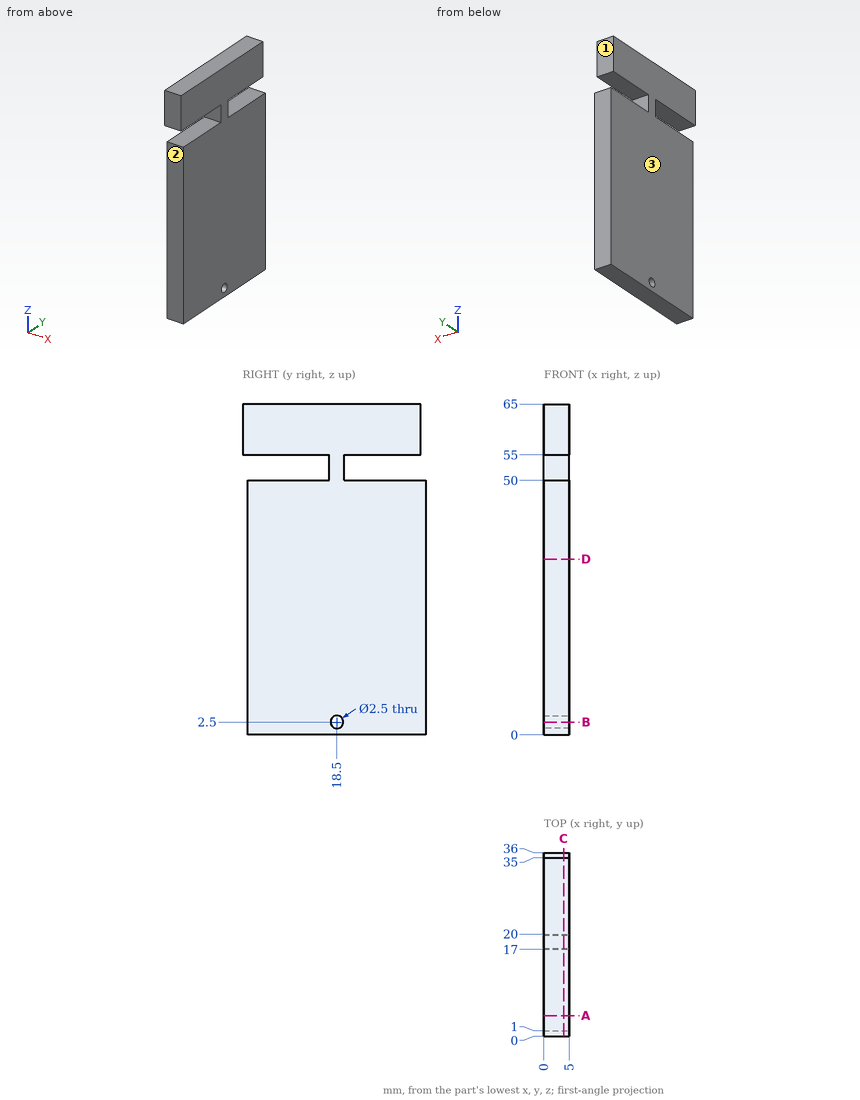
Input: dimensioned drawing with shaded views. Units: mm. Origin: part minimum x, y, z. A direction names the side the tool comes from. Coordinates: 2 decimals unless noted, no trailing zeros. Order: outer loops, then holes, each group sorted by start corner. A loop starts at its lowest first (then second) coordinate and runs counter-clockwise, first axis right, second up. Notation, with made-up numbers: M -21,-35.5 L 38,-35.5 A19 cw 38,-30.5 Z; hole C 35,75 d6. An arc over 180 degrees is marked long. Write each question's results on one line, items separated by ' | '. Start each with the question number.
Item 1: Cut plane D-D (z = 34.5). Return loops of the section in (x, y), and give its area (3 significant figures).
Item 2: Line query: probe 1 along Z at (x, y) = (1.9, 13); probe 2 along Y at (x, z) = (2.95, 2.5); probe 3 along Y at (x, z) = (1.9, 21). Output: solid intervals per line, ascending.
Item 3: Set-up query: the marked faces 1, 2 and 3. Return all of +Z, -Z, +X, -X, +Y, -Y with unobstructed straight access to the full face (end or side cutting, diameter ignored); none if empty.
Item 4: Cut plane B-B (z = 2.5). Return loops of the section in (x, y), and give its area (4 significant figures).
Item 5: Cut plane A-A (y = 4). Return loops of the section in (x, z).
Item 6: First-contact query: pin 1 Ø1.5 at (x, z) = (2.5, 59.5) entering from +Y. Flat tip, straight axial feed; report the tip coordinate or a pass-through.
Item 7: Cut plane C-C (x = 3.9). Return loops of the section in (y, z).
Checked values:
1) outline: M 0,1 L 5,1 L 5,36 L 0,36 Z | area: 175 mm2
2) probe 1: z = 0 to 50, 55 to 65 | probe 2: y = 1 to 17.25, 19.75 to 36 | probe 3: y = 1 to 36
3) face 1: +Z, +X, -X, +Y | face 2: -Z, +X, -X, -Y | face 3: +Z, -Z, -X, +Y, -Y
4) outline: M 0,1 L 5,1 L 5,17.25 L 0,17.25 Z; M 0,19.75 L 5,19.75 L 5,36 L 0,36 Z | area: 162.5 mm2
5) outline: M 0,0 L 5,0 L 5,50 L 0,50 Z; M 0,55 L 5,55 L 5,65 L 0,65 Z
6) pin 1: stops at y = 35
7) outline: M 0,55 L 17,55 L 17,50 L 1,50 L 1,0 L 36,0 L 36,50 L 20,50 L 20,55 L 35,55 L 35,65 L 0,65 Z; hole C 18.5,2.5 d2.5
